Build history of the part. All positions in model axes, mm. Round coordinates to 2 decimals unless told otherwise and drop trailing zeros. Write each loop counter-clockwise with the first axis right and the second up, starting at its lowest first coordinate (ties: lowest second). Pieces come first, ordered by that corner, then holes. Notation, with made-up numbers: M 55,4 L 92,4 A20 ccw 92,25 Z; hole C -18,86.25 d3. An arc over 180 degrees is marked long. Use a Markdown table: item, result.
from build123d import *

# Parameters (mm, degrees)
F0_W     = 100.000004
F0_H     = 88.9
F1_DEPTH = 38.1
F2_SIZE  = 38.1
F4_D     = 7.874


with BuildPart() as f1:
    # F0 (on Top) → F1 (new body)
    with BuildSketch(Plane.XY):
        Rectangle(F0_W, F0_H)
    extrude(amount=F1_DEPTH)

    # F2
    f2_edges = [f1.edges().sort_by_distance(p)[0] for p in [
        (50.000002, 44.45, 19.05),
        (-50.000002, 44.45, 19.05),
    ]]
    chamfer(f2_edges, length=F2_SIZE)

    # F4 (through all)
    with Locations(Plane(origin=(0, 0, 0), x_dir=(1, 0, 0), z_dir=(0, 0, -1))):
        with Locations((-27.775002, 22.225), (27.775002, 22.225)):
            Hole(F4_D / 2)


solid = f1.part
Q1. Drop flat-ended pins along their axis: P1, Ø8, axis at x = -38.5, z = 32.5, coming from the +Y side; P2, Ø10, axis at x = -27.78, y = -22.22, coming from the -Z side; P3, Ø1.5, axis at x = -32.5, z = 27, coming from the +Y side; P4, Ø12, axis at y = 19.5, z = 21, coming from the +X side. Give the stop position or say it passes through.
Response values:
| item | result |
|---|---|
| P1 | stops at y = 21.85 |
| P2 | stops at z = 0 |
| P3 | stops at y = 24.6 |
| P4 | stops at x = 42.85 |
Q2. Cut at B-B on z = 27. Give the cut face in (x, y) (3 decimals), and give its area (3 significant figures).
Response values:
| item | result |
|---|---|
| outline | M -50,-44.45 L 50,-44.45 L 50,6.35 L 11.9,44.45 L -11.9,44.45 L -50,6.35 Z; hole C -27.775,-22.225 d7.874; hole C 27.775,-22.225 d7.874 |
| area | 7,340 mm2 |
Q3. Cut at C-C on y = 39. Give the cut face in (x, z).
Response values:
| item | result |
|---|---|
| outline | M -17.35,0 L 17.35,0 L 17.35,38.1 L -17.35,38.1 Z |
Q4. Cut at A-A on x = -28. Give the cut face in (y, z).
Response values:
| item | result |
|---|---|
| outline | M -44.45,0 L -26.16,0 L -26.16,38.1 L -44.45,38.1 Z; M -18.29,0 L 28.35,0 L 28.35,38.1 L -18.29,38.1 Z |
Q5. Drill centre lines: L1, parallel to X at y = -25.5, z = 28; L2, parallel to X at y = 32.5, z = 25; L3, parallel to X at y = 22.5, z = 20. Where is each one in solid material? Low to high.
Response values:
| item | result |
|---|---|
| L1 | x = -50 to -29.96, -25.59 to 25.59, 29.96 to 50 |
| L2 | x = -23.85 to 23.85 |
| L3 | x = -33.85 to 33.85 |
Q6. Two-plate mould, pull along Y, no slides. Class faces 1 (the cylindrical face through (-26.92, -18.38, 19.32)), 2 (the flat face through (50, -19, 19)), 3 (the flat face through (30.68, 25.67, 18.78)): +Y half, -Y half, draft (parallel to the pull), parting line (faces both ways), or undercut.
Response values:
| item | result |
|---|---|
| face 1 | undercut |
| face 2 | draft |
| face 3 | +Y half |
Q7. Cut at D-D on x = 14. Give the cut face in (y, z).
Response values:
| item | result |
|---|---|
| outline | M -44.45,0 L 42.35,0 L 42.35,38.1 L -44.45,38.1 Z |
